```python
from build123d import *

# Parameters (mm, degrees)
F1_DEPTH  = 15
F2_W      = 30.607
F2_H      = 10
F3_DEPTH  = 25
F4_DEPTH  = 20
F6_DEPTH  = 9
F7_DEPTH  = 9
F8_R      = 11
F9_R      = 2.5
F10_DEPTH = 25


# Not quite as in the source:
# - a feature names something its author has since deleted; it is built from what else it names


with BuildPart() as f1:
    # F0 (on Top) → F1 (new body)
    with BuildSketch(Plane.XY):
        Polygon((37.435, 25.263), (2.828, 25.263), (0, 22.435), (0, 2.828), (2.828, 0), (37.435, 0), (40.263, 2.828), (40.263, 22.435), align=None)
    extrude(amount=F1_DEPTH)

    # F2 (on face) → F3 (cut)
    with BuildSketch(Plane.XZ):
        with Locations((20.1315, 8)):
            Rectangle(F2_W, F2_H)
    extrude(amount=-F3_DEPTH, mode=Mode.SUBTRACT)

    # F2 (on face) → F4 (cut)
    with BuildSketch(Plane.XZ):
        with Locations((20.1315, 8)):
            Rectangle(F2_W, F2_H)
    extrude(amount=-F4_DEPTH, mode=Mode.SUBTRACT)

    # F5 (on face) → F6 (join)
    with BuildSketch(Plane(origin=(0, 0, 0), x_dir=(1, 0, 0), z_dir=(0, 0, -1))):
        with BuildLine():
            ThreePointArc((12.1315, -20.463), (11.1315, -19.463), (10.1315, -20.463))
            Line((10.1315, -20.463), (12.1315, -20.463))
        make_face()
        with BuildLine():
            Line((12.1315, -20.463), (10.1315, -20.463))
            ThreePointArc((10.1315, -20.463), (11.1315, -21.463), (12.1315, -20.463))
        make_face()
        with BuildLine():
            Line((18.6315, -20.463), (21.6315, -20.463))
            ThreePointArc((21.6315, -20.463), (20.1315, -18.963), (18.6315, -20.463))
        make_face()
        with BuildLine():
            ThreePointArc((18.6315, -20.463), (20.1315, -21.963), (21.6315, -20.463))
            Line((21.6315, -20.463), (18.6315, -20.463))
        make_face()
        with BuildLine():
            ThreePointArc((28.1315, -20.463), (29.1315, -21.463), (30.1315, -20.463))
            Line((30.1315, -20.463), (28.1315, -20.463))
        make_face()
        with BuildLine():
            Line((28.1315, -20.463), (30.1315, -20.463))
            ThreePointArc((30.1315, -20.463), (29.1315, -19.463), (28.1315, -20.463))
        make_face()
    extrude(amount=F6_DEPTH)

    # F5 (on face) → F7 (join)
    with BuildSketch(Plane(origin=(0, 0, 0), x_dir=(1, 0, 0), z_dir=(0, 0, -1))):
        with BuildLine():
            Line((19.3815, -4.8), (20.8815, -4.8))
            ThreePointArc((20.8815, -4.8), (20.1315, -4.05), (19.3815, -4.8))
        make_face()
        with BuildLine():
            ThreePointArc((19.3815, -4.8), (20.1315, -5.55), (20.8815, -4.8))
            Line((20.8815, -4.8), (19.3815, -4.8))
        make_face()
    extrude(amount=F7_DEPTH)

    # F8
    f8_edges = [f1.edges().sort_by_distance(p)[0] for p in [
        (40.263, 12.6315, 15),
        (0, 12.6315, 15),
    ]]
    fillet(f8_edges, radius=F8_R)

    # F9 (on face) → F10 (cut)
    with BuildSketch(Plane.XY.offset(3)):
        with Locations((7.828, 12.5)):
            Circle(F9_R)
    extrude(amount=-F10_DEPTH, mode=Mode.SUBTRACT)


solid = f1.part
```
The model under review builds one solid part; all positions refer to its coordinate system, in mm. A direction names the side the tool comes from. Give positions to 0.01 mm unless a question says otherwise; leave off trailing zeros. Write each loop counter-clockwise with the first axis right and the second up, starting at its lowest first coordinate (ties: lowest second). Pieces come first, ordered by that corner, then holes. Notation, with made-up numbers: (-23, 36.25) -> (-14, 36.25) arc R35 ccw to (-14, 74.25) -> close; hole circle Ø10 at (-26, 57.25). An arc over 180 degrees is marked (long way). Answer in a Markdown table with one row per item.
1) Add section D-D on x = 34. State the section outline as (y, z) points, plus the area to 3 significant figures.
Worked answers:
| item | result |
|---|---|
| outline | (0, 0) -> (25.26, 0) -> (25.26, 13.93) -> (0, 13.93) -> (0, 13) -> (25, 13) -> (25, 3) -> (0, 3) -> close |
| area | 102 mm² |
2) Tool access review of faces 5 (the cylindrical face through (10.67, 19.576, -4.437)), 6 (the flat face through (20, 12, 3)), 7 (the cylindrical face through (3.308, 12.455, 11.863)): name each direction out of +Z, -Z, +X, -X, +Y, -Y from which nothing blocks a thin tool from reaching the whole face with its end or side.
Worked answers:
| item | result |
|---|---|
| face 5 | -Z |
| face 6 | -Y |
| face 7 | +Z, -X, +Y, -Y |
3) Add section C-C on y = 12.5. State the section outline as (x, z) points (3 decimals), plus the area to 3 significant figures.
Worked answers:
| item | result |
|---|---|
| outline | (0, 0) -> (5.328, 0) -> (5.328, 3) -> (4.828, 3) -> (4.828, 13) -> (35.435, 13) -> (35.435, 3) -> (10.328, 3) -> (10.328, 0) -> (40.263, 0) -> (40.263, 4) arc R11 ccw to (29.263, 15) -> (11, 15) arc R11 ccw to (0, 4) -> close |
| area | 231 mm² |
4) For L1, parallel to Z at x = 27.5, y = 14.5; L2, parallel to Z at x = 20, y = 20.5; L3, parallel to Y at x = 34, z = 11.75, list the stretches that pass through material, from the lowest coordinate up. Write a range as [from, to].
Worked answers:
| item | result |
|---|---|
| L1 | [0, 3], [13, 15] |
| L2 | [-9, 3], [13, 15] |
| L3 | [25, 25.26] |
5) Add section A-A on y = 6.5. State the section outline as (x, z) points (3 decimals).
Worked answers:
| item | result |
|---|---|
| outline | (0, 0) -> (40.263, 0) -> (40.263, 4) arc R11 ccw to (29.263, 15) -> (11, 15) arc R11 ccw to (0, 4) -> close; hole (4.828, 3) -> (35.435, 3) -> (35.435, 13) -> (4.828, 13) -> close |
6) Mouldability with a two-part tool opening along Y and no side actions: class faces 1 (the cylindrical face through (20.46, 19, -4.44)), 2 (the flat face through (38.829, 1.394, 4.34)), 3 (the flat face through (20, 25.263, 7)), 4 (the cylindrical face through (7.29, 10.06, 1.52)) as +Y half, -Y half, draft (parallel to the pull), parting line (faces both ways), or undercut.
Worked answers:
| item | result |
|---|---|
| face 1 | undercut |
| face 2 | -Y half |
| face 3 | +Y half |
| face 4 | undercut |
7) Clearance check with flat-ended pins moving along their axes: P1, Ø1, axis at y = 4, z = -1, coming from the +X side; P2, Ø1.5, axis at x = 4, y = 20, coming from the -Z side; P3, Ø5, axis at y = 18, z = 10.5, coming from the -X side; P4, Ø3, axis at x = 14.5, z = -2, coming from the -Y side. State where each tip first meets the part, or that it passes through.
Worked answers:
| item | result |
|---|---|
| P1 | x = 20.82 |
| P2 | z = 0 |
| P3 | x = 0.75 |
| P4 | through |
8) Add section B-B on z = 1. State the section outline as (x, y) points (3 decimals), plus the area to 3 significant figures.
Worked answers:
| item | result |
|---|---|
| outline | (0, 2.828) -> (2.828, 0) -> (37.435, 0) -> (40.263, 2.828) -> (40.263, 22.435) -> (37.435, 25.263) -> (2.828, 25.263) -> (0, 22.435) -> close; hole circle Ø5 at (7.828, 12.5) |
| area | 982 mm² |
